```python
from build123d import *

# Parameters (mm, degrees)
SKETCH1_R           = 4.7625
BOSS_EXTRUDE1_DEPTH = 25.4
SKETCH2_W           = 12.7
SKETCH2_H           = 8.89
SKETCH2_H_2         = 18.382780547
CUT_EXTRUDE1_DEPTH  = 64.5
SKETCH3_R           = 3.175
CUT_EXTRUDE2_DEPTH  = 7.35


with BuildPart() as part:
    # Sketch1 → Boss-Extrude1 (new body)
    with BuildSketch(Plane.XY):
        with BuildLine():
            Line((31.75, -8.89), (6.29056934, 13.502227791))
            ThreePointArc((6.29056934, 13.502227791), (0, 15.875), (-6.29056934, 13.502227791))
            Line((-6.29056934, 13.502227791), (-31.75, -8.89))
            Line((-31.75, -8.89), (-31.75, -15.24))
            Line((-31.75, -15.24), (31.75, -15.24))
            Line((31.75, -15.24), (31.75, -8.89))
        make_face()
        with Locations((0, 6.35)):
            Circle(SKETCH1_R, mode=Mode.SUBTRACT)
    extrude(amount=BOSS_EXTRUDE1_DEPTH)

    # Sketch2 → Cut-Extrude1 (cut, through all)
    with BuildSketch(Plane(origin=(31.75, 0, 0), x_dir=(0, 0, -1), z_dir=(1, 0, 0))):
        with Locations((-12.7, -4.445)):
            Rectangle(SKETCH2_W, SKETCH2_H)
        with Locations((-12.7, 9.191390273)):
            Rectangle(SKETCH2_W, SKETCH2_H_2)
    extrude(amount=-CUT_EXTRUDE1_DEPTH, mode=Mode.SUBTRACT)

    # Sketch3 → Cut-Extrude2 (cut, through all)
    with BuildSketch(Plane(origin=(0, -8.89, 0), x_dir=(1, 0, 0), z_dir=(0, 1, 0))):
        with Locations((-19.05, -12.7)):
            Circle(SKETCH3_R)
        with Locations((19.05, -12.7)):
            Circle(SKETCH3_R)
    extrude(amount=-CUT_EXTRUDE2_DEPTH, mode=Mode.SUBTRACT)


solid = part.part
```
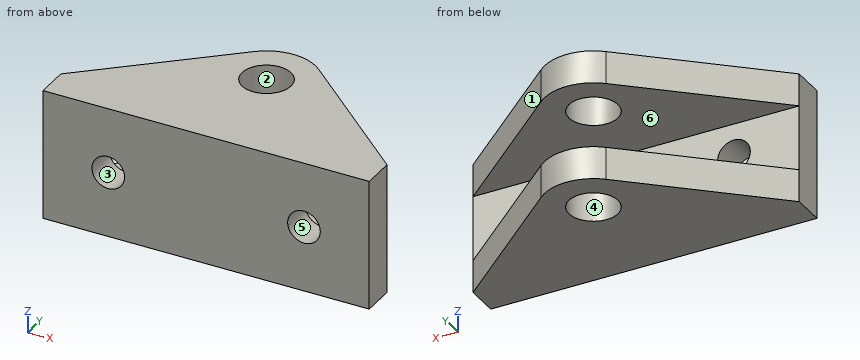
Design review of the part built by this model. Coordinates are the model's own, in mm. Face numbers are marked on the shaded views. A direction names the side the tool comes from. Coordinates: 2 decimals unless noted, no trailing zeros. Order: outer loops, then holes, each group sorted by start corner. A loop starts at its lowest first (then second) coordinate and runs counter-clockwise, first axis right, second up. Notation, with made-up numbers: (29.5, 66.25) -> (74.5, 66.25) arc R25 ccw to (74.5, 100.25) -> close; hole circle Ø4 at (63, -16.75). An arc over 180 degrees is marked (long way). One line per item, written item: value. Start each with the question number.
Q1. Tool access review of the marked faces 5 and 6: name each direction out of +Z, -Z, +X, -X, +Y, -Y from which nothing blocks a thin tool from reaching the whole face with its end or side.
Q2. Insertion check: pin 1 Ø12.5 at (x, y) = (-0.5, 7) entering from -Z; pin 2 Ø3 at (y, z) = (1.5, 20.5) entering from -X; pin 3 Ø4 at (y, z) = (5.5, 21) entering from +X; pin 4 Ø10 at (x, z) = (19.05, 12.7) entering from +Y. Each pin has a flat end and moves straight along its axis. Give the tip position at first contact, or say it passes through.
Q3. Take a section at B-B, the plane x = 19.05. State the section outline as (y, z) points (3 decimals).
Q4. For probe 1 along X at (y, z) = (-13, 12.7) (3 decimals); probe 2 along Z at (x, y) = (-25.5, -5); probe 3 along Y at (x, z) = (0, 2.25) (1 decimal), list the stretches that pass through material, from the lowest coordinate up.
Q5. Take a section at C-C, the plane y = 6.35. State the section outline as (x, z) points.
Q6. Take a section at A-A, the plane z = 12.7. State the section outline as (x, y) points (3 decimals).
Q7. Mouldability with a two-part tool opening along Y and no side actions: class the marked faces 1, 2, 3 and 4 as pulls with the +Y half, pulls with the -Y half, needs draft (parallel to the pull), parting line crosses it, or undercut.
Values follow:
1. face 5: +Y, -Y
1. face 6: +X, -X, +Y
2. pin 1: stops at z = 0
2. pin 2: stops at x = -21.64
2. pin 3: stops at x = 17.66
2. pin 4: stops at y = -8.89
3. outline: (-15.24, 0) -> (2.28, 0) -> (2.28, 6.35) -> (-8.89, 6.35) -> (-8.89, 9.525) -> (-15.24, 9.525) -> close; (-15.24, 15.875) -> (-8.89, 15.875) -> (-8.89, 19.05) -> (2.28, 19.05) -> (2.28, 25.4) -> (-15.24, 25.4) -> close
4. probe 1: x = -31.75 to -22.225, -15.875 to 15.875, 22.225 to 31.75
4. probe 2: z = 0 to 6.35, 19.05 to 25.4
4. probe 3: y = -15.2 to 1.6, 11.1 to 15.9
5. outline: (-14.42, 0) -> (-4.76, 0) -> (-4.76, 6.35) -> (-14.42, 6.35) -> close; (-14.42, 19.05) -> (-4.76, 19.05) -> (-4.76, 25.4) -> (-14.42, 25.4) -> close; (4.76, 0) -> (14.42, 0) -> (14.42, 6.35) -> (4.76, 6.35) -> close; (4.76, 19.05) -> (14.42, 19.05) -> (14.42, 25.4) -> (4.76, 25.4) -> close
6. outline: (-31.75, -15.24) -> (-22.225, -15.24) -> (-22.225, -8.89) -> (-31.75, -8.89) -> close; (-15.875, -15.24) -> (15.875, -15.24) -> (15.875, -8.89) -> (-15.875, -8.89) -> close; (22.225, -15.24) -> (31.75, -15.24) -> (31.75, -8.89) -> (22.225, -8.89) -> close
7. face 1: pulls with the +Y half
7. face 2: undercut
7. face 3: needs draft
7. face 4: undercut
